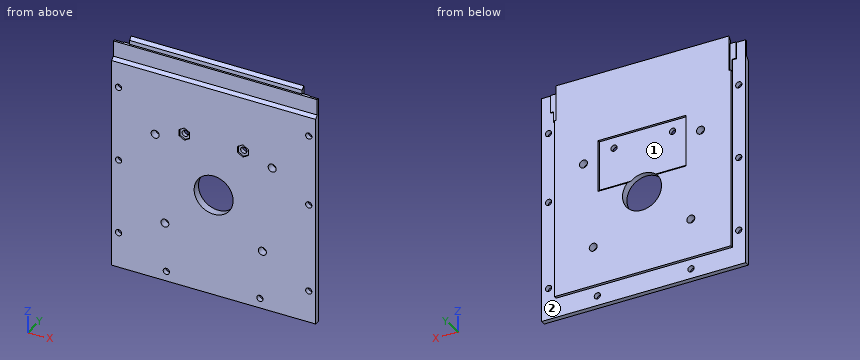
```python
from build123d import *

# Parameters (mm, degrees)
SKETCH_1_W           = 90.5
SKETCH_1_H           = 97
EXTRUDE_1_DEPTH      = 2
SKETCH_2_W           = 104.525
SKETCH_2_H           = 124
SKETCH_2_R           = 1.6
EXTRUDE_2_DEPTH      = 2.5
SKETCH_3_W           = 88.5
SKETCH_3_H           = 17
EXTRUDE_3_DEPTH      = 2
SKETCH_4_W           = 1
SKETCH_4_H           = 5
CUT_EXTRUDE_1_DEPTH  = 2
CUT_EXTRUDE_2_DEPTH  = 150.601890446
SKETCH_6_W           = 45
SKETCH_6_H           = 25
CUT_EXTRUDE_3_DEPTH  = 1.7
CUT_EXTRUDE_4_REACH  = 146.972
SKETCH_7_R           = 1.6
CHAMFER_1_SIZE       = 2
CUT_EXTRUDE_5_REACH  = 147.014
SKETCH_8_R           = 2.05
CUT_EXTRUDE_6_REACH  = 147.014
SKETCH_9_R           = 10
CUT_EXTRUDE_7_DEPTH  = 0.8
CUT_EXTRUDE_8_REACH  = 151.602
SKETCH_11_W          = 6.5
SKETCH_11_H          = 2.5
CHAMFER_2_SIZE       = 2
SKETCH_12_W          = 104.525
SKETCH_12_H          = 9.5
EXTRUDE_4_DEPTH      = 1
SKETCH_13_W          = 2
SKETCH_13_H          = 14.5
EXTRUDE_5_DEPTH      = 0.5
SKETCH_14_W          = 1.5
SKETCH_14_H          = 9
SKETCH_14_W_2        = 1
EXTRUDE_6_DEPTH      = 0.5
SKETCH_15_W          = 88.5
SKETCH_15_H          = 2.828427125
EXTRUDE_7_DEPTH      = 2
CUT_EXTRUDE_9_DEPTH  = 0.5
SKETCH_17_W          = 2
SKETCH_17_H          = 6
CUT_EXTRUDE_10_DEPTH = 0.5


with BuildPart() as part:
    # 草图1 → 凸台-拉伸1 (new body)
    with BuildSketch(Plane(origin=(0, 0, 0), x_dir=(1, 0, 0), z_dir=(0, 1, 0))):
        with Locations((45.25, 48.5)):
            Rectangle(SKETCH_1_W, SKETCH_1_H)
    extrude(amount=EXTRUDE_1_DEPTH)

    # 草图2 → 凸台-拉伸2 (add)
    with BuildSketch(Plane.XZ):
        with Locations((45.5125, -45)):
            Rectangle(SKETCH_2_W, SKETCH_2_H)
        with Locations(Location((21.25, -102, 0), (0, 0, 270))):
            Circle(SKETCH_2_R, mode=Mode.SUBTRACT)
        with Locations(Location((69.25, -102, 0), (0, 0, 270))):
            Circle(SKETCH_2_R, mode=Mode.SUBTRACT)
        with Locations(Location((-3.25, -89, 0), (0, 0, 270))):
            Circle(SKETCH_2_R, mode=Mode.SUBTRACT)
        with Locations(Location((94.275, -90.75, 0), (0, 0, 270))):
            Circle(SKETCH_2_R, mode=Mode.SUBTRACT)
        with Locations(Location((-3.25, -13, 0), (0, 0, 270))):
            Circle(SKETCH_2_R, mode=Mode.SUBTRACT)
        with Locations(Location((-3.25, -51, 0), (0, 0, 270))):
            Circle(SKETCH_2_R, mode=Mode.SUBTRACT)
        with Locations(Location((94.275, -9.75, 0), (0, 0, 270))):
            Circle(SKETCH_2_R, mode=Mode.SUBTRACT)
        with Locations(Location((94.275, -45.75, 0), (0, 0, 270))):
            Circle(SKETCH_2_R, mode=Mode.SUBTRACT)
    extrude(amount=EXTRUDE_2_DEPTH)

    # 草图3 → 凸台-拉伸3 (add)
    with BuildSketch(Plane(origin=(0, 0, 0), x_dir=(1, 0, 0), z_dir=(0, 1, 0))):
        with Locations((45.25, -8.5)):
            Rectangle(SKETCH_3_W, SKETCH_3_H)
    extrude(amount=EXTRUDE_3_DEPTH)

    # 草图4 → 切除-拉伸1 (cut)
    with BuildSketch(Plane(origin=(0, 0, 0), x_dir=(1, 0, 0), z_dir=(0, 1, 0))):
        with Locations((0.5, 2.5)):
            Rectangle(SKETCH_4_W, SKETCH_4_H)
        with Locations((90, 2.5)):
            Rectangle(SKETCH_4_W, SKETCH_4_H)
    extrude(amount=CUT_EXTRUDE_1_DEPTH, mode=Mode.SUBTRACT)

    # 草图5 → 切除-拉伸2 (cut, through all)
    with BuildSketch(Plane(origin=(97.775, 0, 0), x_dir=(0, 0, -1), z_dir=(1, 0, 0))):
        Polygon((-8.5, -2.5), (-8.5, 0), (-9.5, 0), (-11.5, 2), (-17, 2), (-17, -2.5), align=None)
    extrude(amount=-CUT_EXTRUDE_2_DEPTH, mode=Mode.SUBTRACT)

    # 草图6 → 切除-拉伸3 (cut)
    with BuildSketch(Plane(origin=(0, 2, 0), x_dir=(1, 0, 0), z_dir=(0, 1, 0))):
        with Locations((45.5125, 34.5)):
            Rectangle(SKETCH_6_W, SKETCH_6_H)
    extrude(amount=-CUT_EXTRUDE_3_DEPTH, mode=Mode.SUBTRACT)

    # 草图7 → 切除-拉伸4 (cut, up to next)
    with BuildSketch(Plane(origin=(0, 0.3, 0), x_dir=(1, 0, 0), z_dir=(0, 1, 0)), mode=Mode.PRIVATE) as cut_extrude_4_sk1:
        with Locations(Location((30.5125, 27.5, 0), (0, 0, 270))):
            Circle(SKETCH_7_R)
    cut_extrude_4_tool1 = extrude(cut_extrude_4_sk1.sketch, amount=-CUT_EXTRUDE_4_REACH, mode=Mode.PRIVATE) & part.part
    # 草图7 → 切除-拉伸4 (cut, up to next)
    with BuildSketch(Plane(origin=(0, 0.3, 0), x_dir=(1, 0, 0), z_dir=(0, 1, 0)), mode=Mode.PRIVATE) as cut_extrude_4_sk2:
        with Locations(Location((60.5125, 27.5, 0), (0, 0, 270))):
            Circle(SKETCH_7_R)
    cut_extrude_4_tool2 = extrude(cut_extrude_4_sk2.sketch, amount=-CUT_EXTRUDE_4_REACH, mode=Mode.PRIVATE) & part.part
    add(cut_extrude_4_tool1.solids().sort_by_distance((30.5125, 0.3, -27.5))[0], mode=Mode.SUBTRACT)
    add(cut_extrude_4_tool2.solids().sort_by_distance((60.5125, 0.3, -27.5))[0], mode=Mode.SUBTRACT)

    # 倒角1
    # the kernel refuses this chamfer: 2 mm, written as the material it adds along each edge
    # the kernel refuses this chamfer: 2 mm, written as the material it takes off along each edge
    with BuildSketch(Plane(origin=(23.0125, 2, -47), x_dir=(0, 0.027495876610586296, -0.9996219169112968), z_dir=(1, 0, 0))) as chamfer_1_2_piece_1_section:
        Polygon((CHAMFER_1_SIZE * 0.999621916911, -CHAMFER_1_SIZE * 0.0274958766106), (-CHAMFER_1_SIZE * 0.0274958766106, -CHAMFER_1_SIZE * 0.999621916911), (0, 0), align=None)
    chamfer_1_2_piece_1 = extrude(amount=45, mode=Mode.PRIVATE)
    chamfer_1_2_piece_1 = split(chamfer_1_2_piece_1, bisect_by=Plane(origin=(45.5125, 0.3, -47.679710145), z_dir=(0, 1, 0)), keep=Keep.TOP, mode=Mode.PRIVATE)
    add(chamfer_1_2_piece_1, mode=Mode.SUBTRACT)

    # 草图8 → 切除-拉伸5 (cut, up to next)
    with BuildSketch(Plane(origin=(0, 2, 0), x_dir=(1, 0, 0), z_dir=(0, 1, 0)), mode=Mode.PRIVATE) as cut_extrude_5_sk1:
        with Locations(Location((20.5125, 77, 0), (0, 0, 270))):
            Circle(SKETCH_8_R)
    cut_extrude_5_tool1 = extrude(cut_extrude_5_sk1.sketch, amount=-CUT_EXTRUDE_5_REACH, mode=Mode.PRIVATE) & part.part
    # 草图8 → 切除-拉伸5 (cut, up to next)
    with BuildSketch(Plane(origin=(0, 2, 0), x_dir=(1, 0, 0), z_dir=(0, 1, 0)), mode=Mode.PRIVATE) as cut_extrude_5_sk2:
        with Locations(Location((70.5125, 77, 0), (0, 0, 270))):
            Circle(SKETCH_8_R)
    cut_extrude_5_tool2 = extrude(cut_extrude_5_sk2.sketch, amount=-CUT_EXTRUDE_5_REACH, mode=Mode.PRIVATE) & part.part
    # 草图8 → 切除-拉伸5 (cut, up to next)
    with BuildSketch(Plane(origin=(0, 2, 0), x_dir=(1, 0, 0), z_dir=(0, 1, 0)), mode=Mode.PRIVATE) as cut_extrude_5_sk3:
        with Locations(Location((15.5125, 32, 0), (0, 0, 270))):
            Circle(SKETCH_8_R)
    cut_extrude_5_tool3 = extrude(cut_extrude_5_sk3.sketch, amount=-CUT_EXTRUDE_5_REACH, mode=Mode.PRIVATE) & part.part
    # 草图8 → 切除-拉伸5 (cut, up to next)
    with BuildSketch(Plane(origin=(0, 2, 0), x_dir=(1, 0, 0), z_dir=(0, 1, 0)), mode=Mode.PRIVATE) as cut_extrude_5_sk4:
        with Locations(Location((75.5125, 32, 0), (0, 0, 270))):
            Circle(SKETCH_8_R)
    cut_extrude_5_tool4 = extrude(cut_extrude_5_sk4.sketch, amount=-CUT_EXTRUDE_5_REACH, mode=Mode.PRIVATE) & part.part
    add(cut_extrude_5_tool1.solids().sort_by_distance((20.5125, 2, -77))[0], mode=Mode.SUBTRACT)
    add(cut_extrude_5_tool2.solids().sort_by_distance((70.5125, 2, -77))[0], mode=Mode.SUBTRACT)
    add(cut_extrude_5_tool3.solids().sort_by_distance((15.5125, 2, -32))[0], mode=Mode.SUBTRACT)
    add(cut_extrude_5_tool4.solids().sort_by_distance((75.5125, 2, -32))[0], mode=Mode.SUBTRACT)

    # 草图9 → 切除-拉伸6 (cut, up to next)
    with BuildSketch(Plane(origin=(0, 2, 0), x_dir=(1, 0, 0), z_dir=(0, 1, 0)), mode=Mode.PRIVATE) as cut_extrude_6_sk1:
        with Locations(Location((45.5125, 55, 0), (0, 0, 230.353888853))):
            Circle(SKETCH_9_R)
    cut_extrude_6_tool1 = extrude(cut_extrude_6_sk1.sketch, amount=-CUT_EXTRUDE_6_REACH, mode=Mode.PRIVATE) & part.part
    add(cut_extrude_6_tool1.solids().sort_by_distance((45.5125, 2, -55))[0], mode=Mode.SUBTRACT)

    # 草图10 → 切除-拉伸7 (cut)
    with BuildSketch(Plane.XZ.offset(2.5)):
        Polygon((27.7625, -25.91228676), (27.7625, -29.08771324), (30.5125, -30.675426481), (33.2625, -29.08771324), (33.2625, -25.91228676), (30.5125, -24.324573519), align=None)
        Polygon((57.7625, -25.91228676), (57.7625, -29.08771324), (60.5125, -30.675426481), (63.2625, -29.08771324), (63.2625, -25.91228676), (60.5125, -24.324573519), align=None)
    extrude(amount=-CUT_EXTRUDE_7_DEPTH, mode=Mode.SUBTRACT)

    # 草图11 → 切除-拉伸8 (cut, up to next)
    with BuildSketch(Plane(origin=(97.775, 0, 0), x_dir=(0, 0, -1), z_dir=(1, 0, 0)), mode=Mode.PRIVATE) as cut_extrude_8_sk1:
        with Locations((-5.25, -1.25)):
            Rectangle(SKETCH_11_W, SKETCH_11_H)
    cut_extrude_8_tool1 = extrude(cut_extrude_8_sk1.sketch, amount=-CUT_EXTRUDE_8_REACH, mode=Mode.PRIVATE) & part.part
    add(cut_extrude_8_tool1.solids().sort_by_distance((97.775, -1.25, 5.25))[0], mode=Mode.SUBTRACT)

    # 倒角2
    chamfer_2_edges = [part.edges().sort_by_distance(p)[0] for p in [
        (45.5125, -2.5, 2),
    ]]
    chamfer(chamfer_2_edges, length=CHAMFER_2_SIZE)

    # 草图12 → 凸台-拉伸4 (add)
    with BuildSketch(Plane.XZ):
        with Locations((45.5125, 4.75)):
            Rectangle(SKETCH_12_W, SKETCH_12_H)
    extrude(amount=EXTRUDE_4_DEPTH)

    # 草图13 → 凸台-拉伸5 (add)
    with BuildSketch(Plane(origin=(0, 0, 0), x_dir=(1, 0, 0), z_dir=(0, 1, 0))):
        with Locations((0, -2.25)):
            Rectangle(SKETCH_13_W, SKETCH_13_H)
        with Locations((90.5, -2.25)):
            Rectangle(SKETCH_13_W, SKETCH_13_H)
    extrude(amount=EXTRUDE_5_DEPTH)

    # 草图14 → 凸台-拉伸6 (add)
    with BuildSketch(Plane(origin=(0, 0, 0), x_dir=(1, 0, 0), z_dir=(0, 1, 0))):
        with Locations((92.25, -5)):
            Rectangle(SKETCH_14_W, SKETCH_14_H)
        with Locations((-1.5, -5)):
            Rectangle(SKETCH_14_W_2, SKETCH_14_H)
    extrude(amount=EXTRUDE_6_DEPTH)

    # 草图15 → 凸台-拉伸7 (add, along a direction that is not the sketch's normal)
    with BuildSketch(Plane(origin=(0, -4.75, 4.75), x_dir=(1, 0, 0), z_dir=(0, -0.7071067811865501, 0.7071067811865449))):
        with Locations((45.25, 8.131727983)):
            Rectangle(SKETCH_15_W, SKETCH_15_H)
    extrude(amount=EXTRUDE_7_DEPTH, dir=(0, 0, 1))

    # 草图16 → 切除-拉伸9 (cut)
    with BuildSketch(Plane(origin=(0, 2, 0), x_dir=(1, 0, 0), z_dir=(0, 1, 0))):
        Polygon((1, 5), (1, -13.5), (89.5, -13.5), (89.5, 5), (90.5, 5), (90.5, 97), (0, 97), (0, 5), align=None)
    extrude(amount=-CUT_EXTRUDE_9_DEPTH, mode=Mode.SUBTRACT)

    # 草图17 → 切除-拉伸10 (cut)
    with BuildSketch(Plane(origin=(0, 0.5, 0), x_dir=(1, 0, 0), z_dir=(0, 1, 0))):
        with Locations((-1, 2)):
            Rectangle(SKETCH_17_W, SKETCH_17_H)
    extrude(amount=-CUT_EXTRUDE_10_DEPTH, mode=Mode.SUBTRACT)


solid = part.part
```
Input: part model. Units: mm. Frame: model coordinates. Face numbers are marked on the shaded views. Give positions to 0.01 mm unless a question says otherwise; leave off trailing zeros. Order: outer loops, then holes, each group sorted by start corner. A loop starts at its lowest first (then second) coordinate and runs counter-clockwise, first axis right, second up. Notation, with made-up numbers: (6, 89) - (27, 89) arc R30 cw to (27, 114) - close; hole circle Ø8 at (11.25, -36). An arc over 180 degrees is marked (long way). One line per item, written item: value.
1. Cut plane C-C, the plane z = -102. Output: boundary loops of the cut face in (x, y) (3 decimals), and give its area (3 significant figures).
Determined:
outline: (-6.75, -2.5) - (19.65, -2.5) - (19.65, 0) - (-6.75, 0) - close; (22.85, -2.5) - (67.65, -2.5) - (67.65, 0) - (22.85, 0) - close; (70.85, -2.5) - (97.775, -2.5) - (97.775, 0) - (70.85, 0) - close
area: 245 mm2
2. Draft query along Z for the marked faces 1 and 2. Return one class per face: released by +Z, released by -Z, zero draft, split by the parting line, or undercut.
Determined:
face 1: undercut
face 2: zero draft
3. Line query: probe 1 along X at (y, z) = (-1.75, -102) (3 decimals); probe 2 along X at (y, z) = (-1.7, -89) (3 decimals); probe 3 along X at (y, z) = (-1.8, -51) (3 decimals). Output: solid intervals per line, ascending.
Determined:
probe 1: -6.75 to 19.65, 22.85 to 67.65, 70.85 to 97.775
probe 2: -6.75 to -4.85, -1.65 to 97.775
probe 3: -6.75 to -4.85, -1.65 to 36.347, 54.678 to 97.775
4. Cut plane A-A, the plane z = -77. Give the number of separate pieces and of enclosed holes in the cut face, and give its area (3 significant figures).
Determined:
separate pieces: 3
enclosed holes: 0
area: 364 mm2
5. Cut plane B-B, the plane z = -13. Output: boundary loops of the cut face in (x, y) (3 decimals), and give its area (3 significant figures).
Determined:
outline: (-6.75, -2.5) - (-4.85, -2.5) - (-4.85, 0) - (-6.75, 0) - close; (-1.65, -2.5) - (97.775, -2.5) - (97.775, 0) - (90.5, 0) - (90.5, 1.5) - (0, 1.5) - (0, 0) - (-1.65, 0) - close
area: 389 mm2
6. Pin query (flat end, axial travel): pin 1 Ø3 at (x, z) = (-3.25, -51) entering from -Y; pin 2 Ø12.5 at (x, z) = (52.5, -31.5) entering from +Y; pin 3 Ø1.2 at (y, z) = (1, 5) entering from +X; pin 4 Ø5 at (x, z) = (94.275, -9.75) entering from +Y. Return the tip coordinate at first contact, or that it passes through.
Determined:
pin 1: through
pin 2: y = 0.3
pin 3: x = 93
pin 4: y = 0
